```python
from build123d import *

# Parameters (mm, degrees)
SKETCH1_W           = 140
SKETCH1_H           = 80
BOSS_EXTRUDE1_DEPTH = 6
SKETCH2_R           = 1.6
CUT_EXTRUDE1_DEPTH  = 81.845531726
SKETCH3_R           = 3.5
CUT_EXTRUDE2_DEPTH  = 4.5
SKETCH4_W           = 154
SKETCH4_H           = 94
SKETCH4_W_2         = 140
SKETCH4_H_2         = 80
BOSS_EXTRUDE2_DEPTH = 0.7


with BuildPart() as part:
    # Sketch1 → Boss-Extrude1 (new body)
    with BuildSketch(Plane.XY):
        Rectangle(SKETCH1_W, SKETCH1_H)
    extrude(amount=BOSS_EXTRUDE1_DEPTH)

    # Sketch2 → Cut-Extrude1 (cut, through all)
    with BuildSketch(Plane.XY.offset(6)):
        with Locations((-62, 28)):
            Circle(SKETCH2_R)
        with Locations((-47, 28)):
            Circle(SKETCH2_R)
        with Locations((47, 28)):
            Circle(SKETCH2_R)
        with Locations((62, 28)):
            Circle(SKETCH2_R)
        with Locations((47, -28)):
            Circle(SKETCH2_R)
        with Locations((62, -28)):
            Circle(SKETCH2_R)
        with Locations(Location((-62, -28, 0), (0, 0, 180))):
            Circle(SKETCH2_R)
        with Locations(Location((-47, -28, 0), (0, 0, 180))):
            Circle(SKETCH2_R)
    extrude(amount=-CUT_EXTRUDE1_DEPTH, mode=Mode.SUBTRACT)

    # Sketch3 → Cut-Extrude2 (cut)
    with BuildSketch(Plane(origin=(0, 0, 0), x_dir=(-1, 0, 0), z_dir=(0, 0, -1))):
        with Locations((62, 28)):
            Circle(SKETCH3_R)
        with Locations((47, 28)):
            Circle(SKETCH3_R)
        with Locations((-47, 28)):
            Circle(SKETCH3_R)
        with Locations((-62, 28)):
            Circle(SKETCH3_R)
        with Locations((-47, -28)):
            Circle(SKETCH3_R)
        with Locations((-62, -28)):
            Circle(SKETCH3_R)
        with Locations((62, -28)):
            Circle(SKETCH3_R)
        with Locations((47, -28)):
            Circle(SKETCH3_R)
    extrude(amount=-CUT_EXTRUDE2_DEPTH, mode=Mode.SUBTRACT)

    # Sketch4 → Boss-Extrude2 (add)
    with BuildSketch(Plane.XY.offset(6)):
        Rectangle(SKETCH4_W, SKETCH4_H)
        Rectangle(SKETCH4_W_2, SKETCH4_H_2, mode=Mode.SUBTRACT)
    extrude(amount=-BOSS_EXTRUDE2_DEPTH)


solid = part.part
```
Build history of the part. All positions in model axes, mm. A direction names the side the tool comes from. Give positions to 0.01 mm unless a question says otherwise; leave off trailing zeros. Order: outer loops, then holes, each group sorted by start corner. A loop starts at its lowest first (then second) coordinate and runs counter-clockwise, first axis right, second up. Notation, with made-up numbers: M 69,89.5 L 83,89.5 A17 cw 83,118.5 Z; hole C 72,-21 d8. An arc over 180 degrees is marked long. Return JSON: item names as keys, results as strings.
Q1. Band-saw the part on A-A (x = 47). Give the cut face in (y, z).
Answer list:
{"outline": "M -47,5.3 L -40,5.3 L -40,0 L -31.5,0 L -31.5,4.5 L -29.6,4.5 L -29.6,6 L -47,6 Z; M -26.4,4.5 L -24.5,4.5 L -24.5,0 L 24.5,0 L 24.5,4.5 L 26.4,4.5 L 26.4,6 L -26.4,6 Z; M 29.6,4.5 L 31.5,4.5 L 31.5,0 L 40,0 L 40,5.3 L 47,5.3 L 47,6 L 29.6,6 Z"}
Q2. Flat gauge pins, fed straight in: pin 1 (8 mm diameter, centred on x = 47, y = 28, fed in from +Z); pin 2 (1.5 mm diameter, centred on x = 10.5, z = 4.5, fed in from +Y); pin 3 (2.5 mm diameter, centred on x = -12, z = 1.5, fed in from -Y); pin 4 (2 mm diameter, centred on x = -60.5, y = -29.5, fed in from -Z). Where does each tip first touch, or does it go through?
Answer list:
{"pin 1": "stops at z = 6", "pin 2": "stops at y = 40", "pin 3": "stops at y = -40", "pin 4": "stops at z = 4.5"}
Q3. 3-axis set-ups, long thin cutter, end or side, ignore diameter. For faces 1 (the face through (-1, 1, 6)), 2 (the face through (-1, -40, 3)), 3 (the face through (60, -29, 4.5)): which of +Z, -Z, +X, -X, +Y, -Y reach the whole face in a straight line?
Answer list:
{"face 1": "+Z, +X, -X, +Y, -Y", "face 2": "-Z, +X, -X, -Y", "face 3": "-Z"}
Q4. Band-saw the part on C-C (y = -22). Give the cut face in (x, z).
Answer list:
{"outline": "M -77,5.3 L -70,5.3 L -70,0 L 70,0 L 70,5.3 L 77,5.3 L 77,6 L -77,6 Z"}
Q5. Band-saw the part on B-B (z = 2.95). Count the separate pieces of the cut face and the enclosed holes in it, then the cut area to 3 significant figures.
Answer list:
{"separate pieces": "1", "enclosed holes": "8", "area": "10,900 mm^2"}
Q6. Wall check: probe 1 along Y at (x, z) = (-62, 1.3); probe 2 along Y at (x, z) = (62, 4.85); probe 3 along X at (y, z) = (-25, 2.25). Give the ranges that are in metal, low to high. Write a range as from..to.
Answer list:
{"probe 1": "y = -40..-31.5, -24.5..24.5, 31.5..40", "probe 2": "y = -40..-29.6, -26.4..26.4, 29.6..40", "probe 3": "x = -70..-63.8, -60.2..-48.8, -45.2..45.2, 48.8..60.2, 63.8..70"}
Q7. Two-plate mould, pull along X, no slides. Class faces 4 (the face through (-64, -29, 4.5)), 5 (the face through (70, -1, 3)), 6 (the face through (-1, 40, 3)): pulls with the +X half, pulls with the -X half, needs draft (parallel to the pull), parting line crosses it, or undercut.
Answer list:
{"face 4": "undercut", "face 5": "pulls with the +X half", "face 6": "needs draft"}
